from build123d import *

# Parameters (mm, degrees)
EXTRUDE_1_DEPTH          = 10
SKETCH_2_R               = 335.5
EXTRUDE_2_DEPTH          = 196
EXTRUDE_4_DEPTH          = 154.8
SHELL_START              = 10
SHELL_4_OUTLINE_R        = 330.5
SHELL_4_DEPTH            = 191
SHELL_4_2_DEPTH          = 149.8
CUT_EXTRUDE_2_DEPTH      = 196
SKETCH_6_R               = 80
EXTRUDE_6_DEPTH          = 66.8
SKETCH_6_2_R             = 80
EXTRUDE_7_DEPTH          = 123.6
SKETCH_7_R               = 75
CUT_EXTRUDE_3_DEPTH      = 185.4
SKETCH_9_R               = 10
CUT_EXTRUDE_11_DEPTH     = 25
PATTERN_CIRCULAR_1_COUNT = 4
RIB_START                = -5
RIB_1_DEPTH              = 10
PATTERN_CIRCULAR_3_COUNT = 6
SKETCH_13_R              = 48
CUT_EXTRUDE_12_DEPTH     = 657.646057629


# Read off the part's stored shape, not the designer's step: 抽壳4, 筋1
with BuildPart() as part:
    # 草图1 → 凸台-拉伸1 (new body)
    with BuildSketch(Plane(origin=(0, 0, 0), x_dir=(1, 0, 0), z_dir=(0, 1, 0))):
        with BuildLine():
            ThreePointArc((-145.890781066, 423.95), (-171.576116901, 414.221388401), (-196.61755928, 402.938280488))
            Line((-196.61755928, 402.938280488), (-402.938280488, 196.61755928))
            ThreePointArc((-402.938280488, 196.61755928), (-414.221388401, 171.576116901), (-423.95, 145.890781066))
            Line((-423.95, 145.890781066), (-423.95, -145.890781066))
            ThreePointArc((-423.95, -145.890781066), (-414.221388401, -171.576116901), (-402.938280488, -196.61755928))
            Line((-402.938280488, -196.61755928), (-196.61755928, -402.938280488))
            ThreePointArc((-196.61755928, -402.938280488), (-171.576116901, -414.221388401), (-145.890781066, -423.95))
            Line((-145.890781066, -423.95), (145.890781066, -423.95))
            ThreePointArc((145.890781066, -423.95), (171.576116901, -414.221388401), (196.61755928, -402.938280488))
            Line((196.61755928, -402.938280488), (402.938280488, -196.61755928))
            ThreePointArc((402.938280488, -196.61755928), (414.221388401, -171.576116901), (423.95, -145.890781066))
            Line((423.95, -145.890781066), (423.95, 145.890781066))
            ThreePointArc((423.95, 145.890781066), (414.221388401, 171.576116901), (402.938280488, 196.61755928))
            Line((402.938280488, 196.61755928), (196.61755928, 402.938280488))
            ThreePointArc((196.61755928, 402.938280488), (171.576116901, 414.221388401), (145.890781066, 423.95))
            Line((145.890781066, 423.95), (-145.890781066, 423.95))
        make_face()
    extrude(amount=EXTRUDE_1_DEPTH)

    # 草图5 → 切除-拉伸2 (cut)
    with BuildSketch(Plane.XZ.offset(-10)):
        with BuildLine():
            Line((356, -142.5), (292.649961558, -142.5))
            ThreePointArc((292.649961558, -142.5), (-325.5, 0), (292.649961558, 142.5))
            Line((292.649961558, 142.5), (356, 142.5))
            Line((356, 142.5), (356, -142.5))
        make_face()
    extrude(amount=CUT_EXTRUDE_2_DEPTH, mode=Mode.SUBTRACT)


with BuildPart() as body_2:
    # 草图2 → 凸台-拉伸2 (new body)
    with BuildSketch(Plane(origin=(0, 10, 0), x_dir=(1, 0, 0), z_dir=(0, 1, 0))):
        with Locations(Location((0, 0, 0), (0, 0, 270))):
            Circle(SKETCH_2_R)
    extrude(amount=EXTRUDE_2_DEPTH)


with BuildPart() as body_3:
    # 草图3 → 凸台-拉伸4 (new body)
    with BuildSketch(Plane(origin=(0, 10, 0), x_dir=(1, 0, 0), z_dir=(0, 1, 0))):
        with BuildLine():
            Line((366, 152.5), (366, -152.5))
            Line((366, -152.5), (298.83774862, -152.5))
            ThreePointArc((298.83774862, -152.5), (335.5, 0), (298.83774862, 152.5))
            Line((298.83774862, 152.5), (366, 152.5))
        make_face()
    extrude(amount=EXTRUDE_4_DEPTH)


with BuildPart() as body_2_1:
    add(body_2.part)

    # Combine 1: union body 3
    add(body_3.part)

    # 抽壳4 outline → 抽壳4 (cut)
    with BuildSketch(Plane(origin=(0, 0, 0), x_dir=(1, 0, 0), z_dir=(0, 1, 0)).offset(SHELL_START)):
        Circle(SHELL_4_OUTLINE_R)
    extrude(amount=SHELL_4_DEPTH, mode=Mode.SUBTRACT)

    # Shell 4 2 outline → Shell 4 2 (cut)
    with BuildSketch(Plane(origin=(0, 0, 0), x_dir=(1, 0, 0), z_dir=(0, 1, 0)).offset(SHELL_START)):
        with BuildLine():
            ThreePointArc((295.760037869, 147.5), (330.5, 0), (295.760037869, -147.5))
            Line((295.760037869, -147.5), (361, -147.5))
            Line((361, -147.5), (361, 147.5))
            Line((361, 147.5), (295.760037869, 147.5))
        make_face()
    extrude(amount=SHELL_4_2_DEPTH, mode=Mode.SUBTRACT)

    # Combine 2: union part
    add(part.part)

    # 草图6 → 凸台-拉伸6 (add)
    with BuildSketch(Plane.XZ.offset(-201)):
        with Locations(Location((0, 0, 0), (0, 0, 90))):
            Circle(SKETCH_6_R)
    extrude(amount=-EXTRUDE_6_DEPTH)

    # 草图6<2> → 凸台-拉伸7 (add)
    with BuildSketch(Plane.XZ.offset(-201)):
        with Locations(Location((0, 0, 0), (0, 0, 90))):
            Circle(SKETCH_6_2_R)
    extrude(amount=EXTRUDE_7_DEPTH)

    # 草图7 → 切除-拉伸3 (cut)
    with BuildSketch(Plane.XZ.offset(-77.4)):
        with Locations(Location((0, 0, 0), (0, 0, 270))):
            Circle(SKETCH_7_R)
    extrude(amount=-CUT_EXTRUDE_3_DEPTH, mode=Mode.SUBTRACT)

    # 草图9 → 切除-拉伸11 (cut)
    with BuildSketch(Plane.XZ):
        with Locations(Location((-308.701607463, 231.061282888, 0), (0, 0, 270))):
            Circle(SKETCH_9_R)
        with Locations(Location((-231.061282888, 308.701607463, 0), (0, 0, 270))):
            Circle(SKETCH_9_R)
    cut_extrude_11 = extrude(amount=-CUT_EXTRUDE_11_DEPTH, mode=Mode.SUBTRACT)

    # 阵列(圆周)1: 切除-拉伸11 ×4 about axis
    pattern_circular_1_axis = Axis((0, 0, 0), (0, 1, 0))
    for i in range(1, PATTERN_CIRCULAR_1_COUNT):
        add(cut_extrude_11.rotate(pattern_circular_1_axis, i * 360 / PATTERN_CIRCULAR_1_COUNT), mode=Mode.SUBTRACT)

    # 筋1 outline → 筋1 (add)
    with BuildSketch(Plane.XY.offset(RIB_START)):
        Polygon((-330.5, 104.315910213), (-79.843597113, 82.38631652), (-78, 82.225022673), (-78, 201), (-332, 201), (-332, 104.447143208), align=None)
    rib_1 = extrude(amount=RIB_1_DEPTH)

    # 阵列(圆周)3: 筋1 ×6 about axis, 1 skipped
    pattern_circular_3_axis = Axis((0, 0, 0), (0, 1, 0))
    add([rib_1.rotate(pattern_circular_3_axis, i * 360 / PATTERN_CIRCULAR_3_COUNT) for i in range(1, PATTERN_CIRCULAR_3_COUNT) if i not in (3,)])

    # 草图13 → 切除-拉伸12 (cut, through all)
    with BuildSketch(Plane(origin=(0, 267.8, 0), x_dir=(1, 0, 0), z_dir=(0, 1, 0))):
        with Locations(Location((0, 0, 0), (0, 0, 270))):
            Circle(SKETCH_13_R)
    extrude(amount=-CUT_EXTRUDE_12_DEPTH, mode=Mode.SUBTRACT)


solid = body_2_1.part
Check sheet for the modelled part. Datum: model origin and axes. Units: mm. A direction names the side the tool comes from. Round coordinates to 2 decimals unless told otherwise and drop trailing zeros. Order: outer loops, then holes, each group sorted by start corner. A loop starts at its lowest first (then second) coordinate and runs counter-clockwise, first axis right, second up. Notation, with made-up numbers: M 87.25,0 L 136.25,0 A18 ccw 136.25,24 Z; hole C 58,51 d4. An arc over 180 degrees is marked long. One line per item, written item: value. Start each with the question number.
1. Section check C-C on x = 275. Enter the section's corners in (y, z).
2. Scan lines: line 1 along X through (y, z) = (183, 0); line 2 along X through (y, z) = (125, 0); line 3 along X through (y, z) = (151.5, 50.5). Record each from-to range of solid material in increasing order.
3. Access from +Z, -Z, +X, -X, +Y, -Y to the whole of each face (thin tool, end or side, straight path). Record for faces 1 (the flat face through (342, 159.8, -2)), 2 (the flat face through (366, 86, -2)), 3 (the flat face through (-71.5, 77.4, 23.3)).
4. Section check B-B on y = 131.5. Give the number of separate pieces and of enclosed holes in the cut face, and give its area (3 significant figures).
5. Gauge pin test, flat ends, axial feed: P1, Ø1.5, axis at y = 101, z = 283.5, coming from the -X side; P2, Ø6, axis at x = 19, z = -101.5, coming from the +Y side; P3, Ø1.5, axis at x = 47.5, y = 188.5, coming from the -Z side; P4, Ø18, axis at x = -231.06, z = -308.7, coming from the +Y side. Record the tip position at first contact, or that the pin passes through.
6. Section check D-D on y = 216. Enter the section's corners in (x, z), and give its area (3 significant figures).
7. Release check for a two-part mould opening along Y. For faces 4 (the flat face through (34.4, 267.8, 34.4)), 5 (the cylindrical face through (14.418, 265.335, 45.783)), 6 (the cylindrical face through (-330.18, 104.16, -14.53)), 7 (the flat face through (329, 84, -147.5)) record: released by +Y, released by -Y, zero draft, split by the parting line, or undercut.
Results found:
1. outline: M 0,-324.56 L 10,-324.56 L 10,-192.19 L 206,-192.19 L 206,192.19 L 10,192.19 L 10,324.56 L 0,324.56 L 0,174.14 L 10,174.14 L 10,183.32 L 201,183.32 L 201,-183.32 L 10,-183.32 L 10,-174.14 L 0,-174.14 Z
2. line 1: -335.5 to -75, 75 to 80, 330.5 to 335.5
2. line 2: -335.5 to -75, 75 to 80, 361 to 366
2. line 3: -331.68 to -326.62, -62.05 to -55.45, 55.45 to 62.05, 361 to 366
3. face 1: none
3. face 2: +Z, -Z, +X, +Y
3. face 3: -Y
4. separate pieces: 1
4. enclosed holes: 6
4. area: 26,000 mm^2
5. P1: x = -180.59
5. P2: y = 206
5. P3: z = -332.23
5. P4: through
6. outline: C 0,0 d160; hole C 0,0 d150
6. area: 2,430 mm^2
7. face 4: released by +Y
7. face 5: zero draft
7. face 6: undercut
7. face 7: undercut
